from build123d import *

# Parameters (mm, degrees)
ESBO_O1_W                  = 13.6
ESBO_O1_H                  = 8.3
RESSALTO_EXTRUS_O1_DEPTH   = 18.7
CORTE_EXTRUS_O1_DEPTH      = 21.326153104
CORTE_EXTRUS_O1_DEPTH_BACK = 18.1
ESBO_O4_W                  = 13
ESBO_O4_H                  = 8
CORTE_EXTRUS_O2_REACH      = 22.326
ESBO_O5_R                  = 1.4


with BuildPart() as part:
    # Esboço1 → Ressalto-extrusão1 (new body)
    with BuildSketch(Plane.XY):
        Rectangle(ESBO_O1_W, ESBO_O1_H)
    extrude(amount=RESSALTO_EXTRUS_O1_DEPTH)

    # Esboço4 → Corte-extrusão1 (cut, two sides: drawn at the far end of the back side and taken through both)
    with BuildSketch(Plane.XY.offset(18.7).offset(-CORTE_EXTRUS_O1_DEPTH_BACK)):
        with Locations((0, -0.15)):
            Rectangle(ESBO_O4_W, ESBO_O4_H)
    extrude(amount=CORTE_EXTRUS_O1_DEPTH + CORTE_EXTRUS_O1_DEPTH_BACK, mode=Mode.SUBTRACT)

    # Esboço5 → Corte-extrusão2 (cut, up to next)
    with BuildSketch(Plane(origin=(0, 0, 0), x_dir=(-1, 0, 0), z_dir=(0, 0, -1)), mode=Mode.PRIVATE) as corte_extrus_o2_sk1:
        Circle(ESBO_O5_R)
    corte_extrus_o2_tool1 = extrude(corte_extrus_o2_sk1.sketch, amount=-CORTE_EXTRUS_O2_REACH, mode=Mode.PRIVATE) & part.part
    add(corte_extrus_o2_tool1.solids().sort_by_distance((0, 0, 0))[0], mode=Mode.SUBTRACT)


solid = part.part
Geometry check sheet. Reference: the model listing, model coordinates, mm. A direction names the side the tool comes from. Round coordinates to 2 decimals unless told otherwise and drop trailing zeros. Loops run counter-clockwise (first coordinate to the right, second up) from the corner with the lowest first, then second, coordinate; pieces in that order, holes last.
Item 1: Cross-section at D-D on x = -2.25. Record the boundary of the cut face in (y, z), then the cut area to 3 significant figures.
Item 2: Thickness scan on line 1 (X direction, y = -1, z = 3.25); line 2 (Y direction, x = 0, z = 0.4); line 3 (Z direction, x = 1.5, y = -0.75). Record the ranges inside material, lowest first.
Item 3: Cross-section at A-A on x = 0. Record the boundary of the cut face in (y, z).
Item 4: Access from +Z, -Z, +X, -X, +Y, -Y to the whole of each face (thin tool, end or side, straight path). Record for faces 1 (the flat face through (0, 4.15, 9)), 2 (the flat face through (0, 3.85, 10)).
Item 5: Cross-section at C-C on y = 3. Record the boundary of the cut face in (x, z).
Item 6: Gauge pin test, flat ends, axial feed: pin 1 (3.5 mm diameter, centred on x = 0, y = 0, fed in from +Z); pin 2 (4 mm diameter, centred on x = -0.5, z = 7.5, fed in from -Y). Record the tip position at first contact, or that the pin passes through.
Item 7: Cross-section at B-B on z = 4.75. Record the boundary of the cut face in (x, y), then the cut area to 3 significant figures.
Item 8: Mould release check, pull along X, two halves, no side actions. Record for faces 3 (the flat face through (0, -4.15, 0.3)), 4 (the flat face through (-2, 0, 0.6)), 5 (the flat face through (-6.8, 0, 9)): pulls with the +X half, pulls with the -X half, needs draft (parallel to the pull), parting line crosses it, or undercut.
Answer sheet:
1. outline: (-4.15, 0) - (4.15, 0) - (4.15, 18.7) - (3.85, 18.7) - (3.85, 0.6) - (-4.15, 0.6) - close
1. area: 10.4 mm2
2. line 1: x = -6.8 to -6.5, 6.5 to 6.8
2. line 2: y = -4.15 to -1.4, 1.4 to 4.15
2. line 3: z = 0 to 0.6
3. outline: (-4.15, 0) - (-1.4, 0) - (-1.4, 0.6) - (-4.15, 0.6) - close; (1.4, 0) - (4.15, 0) - (4.15, 18.7) - (3.85, 18.7) - (3.85, 0.6) - (1.4, 0.6) - close
4. face 1: +Z, -Z, +X, -X, +Y
4. face 2: +Z, -Y
5. outline: (-6.8, 0) - (6.8, 0) - (6.8, 18.7) - (6.5, 18.7) - (6.5, 0.6) - (-6.5, 0.6) - (-6.5, 18.7) - (-6.8, 18.7) - close
6. pin 1: stops at z = 0.6
6. pin 2: stops at y = 3.85
7. outline: (-6.8, -4.15) - (-6.5, -4.15) - (-6.5, 3.85) - (6.5, 3.85) - (6.5, -4.15) - (6.8, -4.15) - (6.8, 4.15) - (-6.8, 4.15) - close
7. area: 8.88 mm2
8. face 3: needs draft
8. face 4: undercut
8. face 5: pulls with the -X half
